from build123d import *

# Parameters (mm, degrees)
FILLET1_R          = 0.5
CUT_EXTRUDE1_DEPTH = 10


with BuildPart() as part:
    # Sketch1 → Revolve1 (revolve)
    with BuildSketch(Plane(origin=(0, 0, 0), x_dir=(1, 0, 0), z_dir=(0, 1, 0)), mode=Mode.PRIVATE) as revolve1_sk:
        Polygon((-29.558969675, -16.48093475), (72.441030325, -16.48093475), (72.441030325, -14.98093475), (57.441030325, -14.98093475), (57.441030325, -13.48093475), (-14.558969675, -13.48093475), (-14.558969675, -14.98093475), (-29.558969675, -14.98093475), align=None)
    revolve(revolve1_sk.sketch.rotate(Axis((-29.558969675, 0, 16.48093475), (1, 0, 0)), 180), axis=Axis((-29.558969675, 0, 16.48093475), (1, 0, 0)))

    # Fillet1
    fillet1_edges = [part.edges().sort_by_distance(p)[0] for p in [
        (57.441030325, 0, 14.98093475),
        (-14.558969675, 0, 14.98093475),
    ]]
    fillet(fillet1_edges, radius=FILLET1_R)

    # Sketch2 → Cut-Extrude1 (cut)
    with BuildSketch(Plane.ZY.offset(29.558969675)):
        with BuildLine():
            Line((15.362900761, 1), (17.598968739, 1))
            ThreePointArc((17.598968739, 1), (16.48093475, 1.5), (15.362900761, 1))
        make_face()
    extrude(amount=-CUT_EXTRUDE1_DEPTH, mode=Mode.SUBTRACT)


solid = part.part
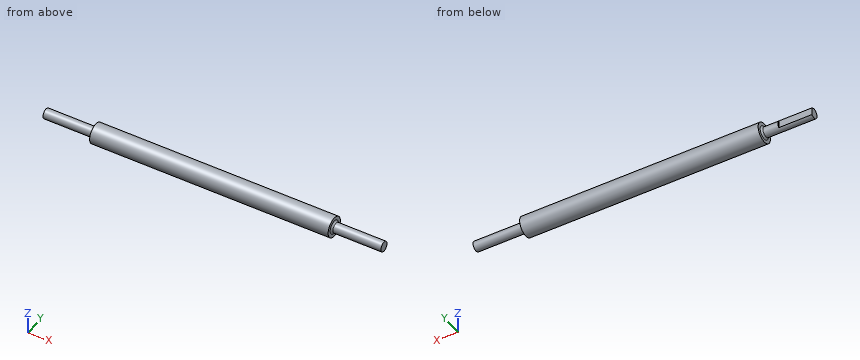
Geometry check sheet. Reference: the model listing, model coordinates, mm. Round coordinates to 2 decimals unless told otherwise and drop trailing zeros. Order: outer loops, then holes, each group sorted by start corner. A loop starts at its lowest first (then second) coordinate and runs counter-clockwise, first axis right, second up. Notation, with made-up numbers: M 7,-10 L 31,-10 A16 cw 31,-5 Z; hole C 81.25,-11.75 d1. An arc over 180 degrees is marked long. Write each question's results on one line, items separated by ' | '. Start each with the question number.
1. Go/stop test with flat-tipped pins: P1, Ø0.6, axis at y = 1.5, z = 16.5, coming from the -X side; P2, Ø1.5, axis at x = 51, y = 1, coming from the -Z side; P3, Ø1.5, axis at y = -0.5, z = 15, coming from the +X side; P4, Ø1.1, axis at x = -26, z = 17, coming from the +Y side. Record where each tip stops, or that it passes through.
2. Cross-section at B-B on x = 18.5. Record the boundary of the cut face in (y, z).
3. Material ranges on L1, parallel to Z at x = 19, y = -0.1; L2, parallel to X at y = -1.3, z = 18.75; L3, parallel to Y at x = 60, z = 16.05, recorded low to high. Write a range as from..to.
4. Cross-section at A-A on y = 0. Record the boundary of the cut face in (x, z).
Resolved:
1) P1: x = -19.56 | P2: z = 13.49 | P3: x = 72.44 | P4: y = 1
2) outline: C 0,16.48 d6
3) L1: 13.48..19.48 | L2: -14.56..57.44 | L3: -1.44..1.44
4) outline: M -29.56,14.98 L -15.06,14.98 A0.5 cw -14.56,14.48 L -14.56,13.48 L 57.44,13.48 L 57.44,14.48 A0.5 cw 57.94,14.98 L 72.44,14.98 L 72.44,17.98 L 57.94,17.98 A0.5 cw 57.44,18.48 L 57.44,19.48 L -14.56,19.48 L -14.56,18.48 A0.5 cw -15.06,17.98 L -29.56,17.98 Z
